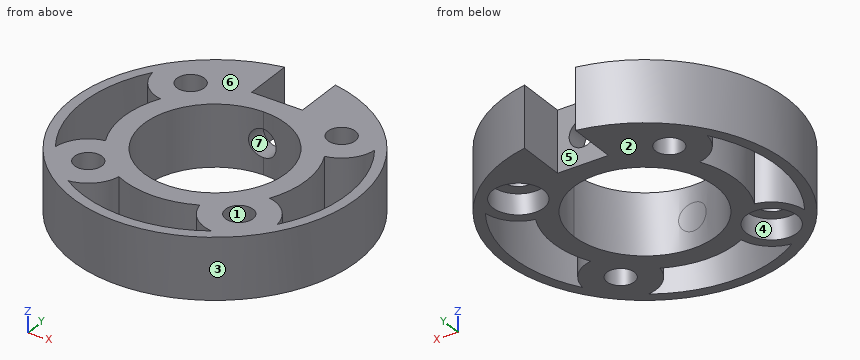
```python
from build123d import *

# Parameters (mm, degrees)
F0_R            = 2.15265
F1_DEPTH        = 9.525
F2_R            = 2.15265
F3_REACH        = 42.6021136501
F5_R            = 3.96875
F6_DEPTH        = 3.175
F8_DEPTH        = 9.525
F8_COPIES_COUNT = 3
F8_COPIES_ANGLE = 180


# Not quite as in the source:
# - a pattern or mirror of a feature is missing from the dataset's text; its kind, count and spacing are read off the source's solid


with BuildPart() as f1:
    # F0 (on Top) → F1 (new body)
    with BuildSketch(Plane.XY):
        with BuildLine():
            Line((3.96875, 14.2875), (0, 14.2875))
            Line((0, 14.2875), (-3.96875, 14.2875))
            Line((-3.96875, 14.2875), (-3.96875, 21.8677764859))
            ThreePointArc((-3.96875, 21.8677764859), (0, -22.225), (3.96875, 21.8677764859))
            Line((3.96875, 21.8677764859), (3.96875, 14.2875))
        make_face()
        with Locations((-11.7865861589, -11.7865861589)):
            Circle(F0_R, mode=Mode.SUBTRACT)
        with Locations((11.7865861589, -11.7865861589)):
            Circle(F0_R, mode=Mode.SUBTRACT)
        with Locations((-11.7865861589, 11.7865861589)):
            Circle(F0_R, mode=Mode.SUBTRACT)
        with BuildLine():
            ThreePointArc((0, 11.1125), (7.8577241059, 7.8577241059), (11.1125, 0))
            ThreePointArc((11.1125, 0), (-7.8577241059, -7.8577241059), (0, 11.1125))
        make_face(mode=Mode.SUBTRACT)
        with Locations((11.7865861589, 11.7865861589)):
            Circle(F0_R, mode=Mode.SUBTRACT)
    extrude(amount=F1_DEPTH)

    f3_end = f1.faces().sort_by_distance((0, -11.1125, 4.7625))[0]
    # F2 (on face) → F3 (cut, up to a face of the model that its end follows)
    with BuildSketch(Plane(origin=(0, 14.2875, 0), x_dir=(-1, 0, 0), z_dir=(0, 1, 0))):
        with Locations((0, 4.7625)):
            Circle(F2_R)
    f3_long = extrude(amount=-F3_REACH, mode=Mode.PRIVATE)
    add(split(f3_long, bisect_by=f3_end, keep=Keep.ALL, mode=Mode.PRIVATE).solids().sort_by_distance((0, 14.2875, 4.7625))[0], mode=Mode.SUBTRACT)

    # F5 (on face) → F6 (cut, through all)
    with BuildSketch(Plane(origin=(0, 0, 0), x_dir=(1, 0, 0), z_dir=(0, 0, -1))):
        with Locations((11.7865861589, -11.7865861589)):
            Circle(F5_R)
        with Locations((-11.7865861589, 11.7865861589)):
            Circle(F5_R)
    extrude(amount=-F6_DEPTH, mode=Mode.SUBTRACT)

    # F7 (on face) → F8 (cut, through all)
    with BuildSketch(Plane(origin=(0, 0, 0), x_dir=(1, 0, 0), z_dir=(0, 0, -1))):
        with BuildLine():
            ThreePointArc((-17.3148424047, -11.229543123), (-15.8788163052, -8.0281867), (-12.8109235396, -6.3255746232))
            ThreePointArc((-12.8109235396, -6.3255746232), (-14.2875, 0), (-12.8109235396, 6.3255746232))
            ThreePointArc((-12.8109235396, 6.3255746232), (-15.8788163052, 8.0281867), (-17.3148424047, 11.229543123))
            ThreePointArc((-17.3148424047, 11.229543123), (-20.6375, 0), (-17.3148424047, -11.229543123))
        make_face()
    f8 = extrude(amount=-F8_DEPTH, mode=Mode.SUBTRACT)

    # F8_copies: F8 ×3 about axis
    f8_copies_axis = Axis((0, 0, 0), (0, 0, 1))
    for i in range(1, F8_COPIES_COUNT):
        add(f8.rotate(f8_copies_axis, i * F8_COPIES_ANGLE / (F8_COPIES_COUNT - 1)), mode=Mode.SUBTRACT)


solid = f1.part
```
Could you check a few things on this model? Use its own coordinates, in mm. Face numbers are marked on the shaded views. A direction names the side the tool comes from. Round coordinates to 2 decimals unless told otherwise and drop trailing zeros. Write each loop counter-clockwise with the first axis right and the second up, starting at its lowest first coordinate (ties: lowest second). Pieces come first, ordered by that corner, then holes. Notation, with made-up numbers: M -6.5,44.5 L 41.5,44.5 A24 ccw 41.5,82.5 Z; hole C 28.5,-24.5 d7. An arc over 180 degrees is marked long. Write each question's results on one line, items separated by ' | '. Start each with the question number.
1. Imagine slicing it at C-C on z = 4. Count the separate pieces of the cut face and the enclosed holes in it, and give its area (3 significant figures).
2. I need wall thicknesses on L1, parallel to Y at x = 4, z = 8.25; L2, parallel to X at y = 13, z = 3; L3, parallel to Y at x = 3.5, z = 3. Which ranges of each line are inside material? Lowest first, please. Write a range as from..to.
3. Imagine slicing it at A-A on y = -8.5. List the corners of the cut face in (x, z) for me (3 decimals).
4. On a 3-axis mill with a long thin cutter (end or side, diameter ignored), from which of +Z, -Z, +X, -X, +Y, -Y can I reach the whole of each face in a straight line? I mean the marked faces 4, 5, 6 and 7. Say none if no direction works.
5. Thinking about a two-plate mould opening in X: for the marked faces 1, 2 and 3, which applies, +X half, -X half, draft (parallel to the pull), parting line (faces both ways), or undercut?
6. I'm going to push flat-ended pins straight in: pin 1 Ø5.5 at (x, z) = (0, 4.76) entering from +Y; pin 2 Ø1 at (x, z) = (-10.5, 2.5) entering from +Y; pin 3 Ø2 at (x, z) = (15.5, 2.5) entering from -Y; pin 4 Ø2.5 at (x, y) = (11.79, -11.79) entering from +Z. Where does each tip first touch, or does it pass through?
7. Imagine slicing it at B-B on x = -8.5. List the corners of the cut face in (y, z) for me (3 decimals).
Result sheet:
1) separate pieces: 1 | enclosed holes: 7 | area: 709 mm^2
2) L1: y = -21.86..-20.25, -13.72..-10.37, 10.37..21.86 | L2: x = -18.03..-13.56, -10.01..-1.24, 1.24..8.01, 15.57..18.03 | L3: y = -21.95..-20.34, -13.85..-10.55, 10.55..14.29
3) outline: M -20.535,0 L -18.806,0 L -18.806,9.525 L -20.535,9.525 Z; M -16.267,0 L -14.011,0 L -14.011,3.175 L -9.562,3.175 L -9.562,0 L -7.158,0 L -7.158,9.525 L -16.267,9.525 Z; M 7.158,0 L 16.267,0 L 16.267,9.525 L 7.158,9.525 Z; M 18.806,0 L 20.535,0 L 20.535,9.525 L 18.806,9.525 Z
4) face 4: -Z | face 5: +Z, -Z, +Y | face 6: +Z, +X, -X, +Y, -Y | face 7: +Y
5) face 1: undercut | face 2: draft | face 3: parting line
6) pin 1: stops at y = 14.29 | pin 2: stops at y = 19.85 | pin 3: stops at y = -16.84 | pin 4: passes through
7) outline: M -20.535,0 L -18.806,0 L -18.806,9.525 L -20.535,9.525 Z; M -16.267,0 L -14.011,0 L -14.011,3.175 L -9.562,3.175 L -9.562,0 L -7.158,0 L -7.158,9.525 L -16.267,9.525 Z; M 7.158,0 L 20.535,0 L 20.535,9.525 L 7.158,9.525 Z
